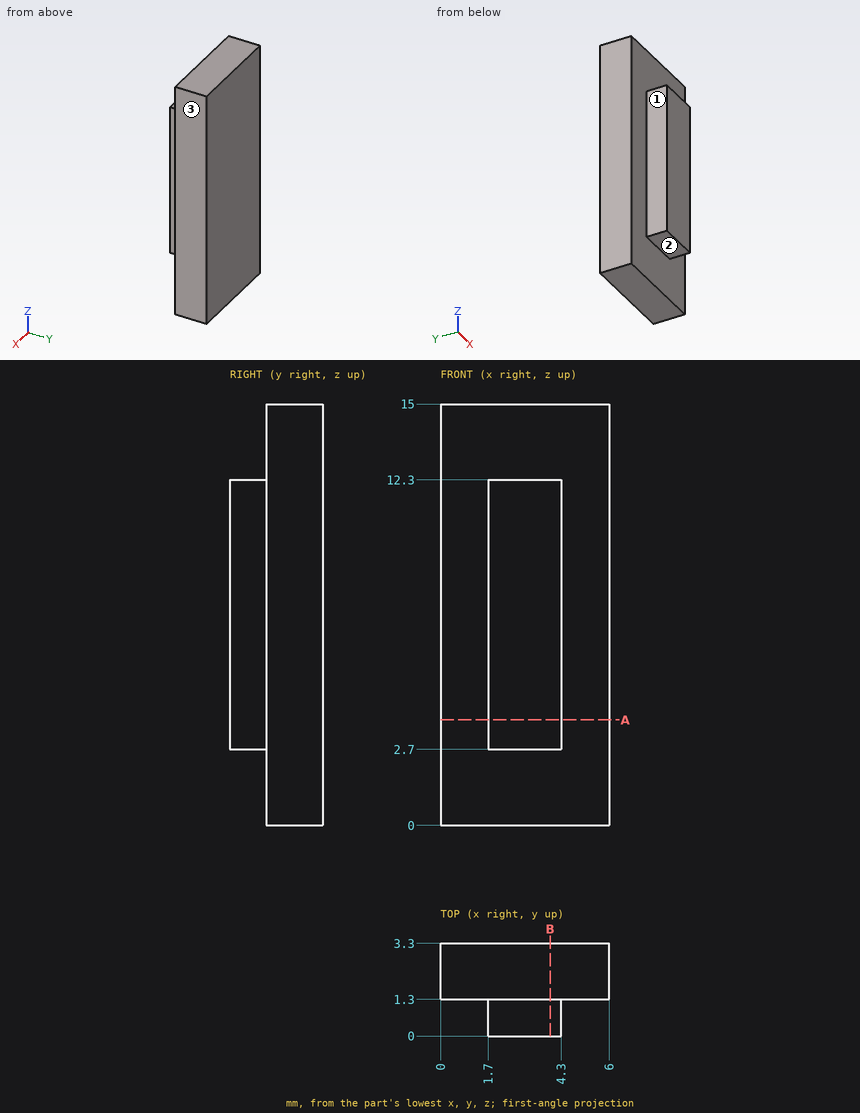
Answer from the drawing. Dimensions are ordinates in mm from the lowest x, y and z of the part. A direction names the side the tool comes from. Give positions to 0.01 mm unless a question says otherwise; leave off trailing zeros. Loops run counter-clockwise (first coordinate to the right, second up) from the corner with the lowest first, then second, coordinate; pieces in that order, holes last.
Item 1: A tool of negligible diameter and unlimited length cuts with its end or side. For the marked faces 1, 2 and 3, from which of +Z, -Z, +X, -X, +Y, -Y can it reach the whole face along a straight path? Write none if from no direction.
Derived:
face 1: +Z, -Z, -X, -Y
face 2: -Z, +X, -X, -Y
face 3: +Z, -Z, +X, +Y, -Y
Item 2: A cutting plane is placed at A-A (z = 3.75). Give the vertices of the cut face in (x, y).
Derived:
outline: (0, 1.3) - (1.7, 1.3) - (1.7, 0) - (4.3, 0) - (4.3, 1.3) - (6, 1.3) - (6, 3.3) - (0, 3.3) - close
Item 3: A cutting plane is placed at B-B (x = 3.9). Give the vertices of the cut face in (y, z).
Derived:
outline: (0, 2.7) - (1.3, 2.7) - (1.3, 0) - (3.3, 0) - (3.3, 15) - (1.3, 15) - (1.3, 12.3) - (0, 12.3) - close
Item 4: Find the intervals of material crossed by line 1 along Y through (x, z) = (4.1, 14.25); line 2 along Z through (x, y) = (4.05, 0.5); line 3 along X through (y, z) = (0.5, 10.5), in increasing order.
Derived:
line 1: y = 1.3 to 3.3
line 2: z = 2.7 to 12.3
line 3: x = 1.7 to 4.3
Item 5: Each of these flat-tipped pins is pushed along its axis until it touches: pin 1 Ø0.6 at (y, z) = (0.5, 8.5) entering from +X; pin 2 Ø0.6 at (x, y) = (3, 0.5) entering from +Z; pin 3 Ø0.6 at (y, z) = (0.5, 5) entering from -X. Where does it stop, or does it pass through?
Derived:
pin 1: stops at x = 4.3
pin 2: stops at z = 12.3
pin 3: stops at x = 1.7
